CAD build for the part. Positions are in the model's coordinates, mm. A direction names the side the tool comes from. Round coordinates to 2 decimals unless told otherwise and drop trailing zeros. Write each loop counter-clockwise with the first axis right and the second up, starting at its lowest first coordinate (ties: lowest second). Pieces come first, ordered by that corner, then holes. Notation, with made-up numbers: (7.5, -27) -> (45.5, -27) arc R9 ccw to (45.5, -22) -> close; hole circle Ø4 at (-17, -33). An arc over 180 degrees is marked (long way). Put each result on its own line as item: value. Start each with the question number.
1. 3-axis set-ups, long thin cutter, end or side, ignore diameter. For faces 1 (the flat face through (10, -8, 1)), 2 (the flat face through (-10, 8, 1)), 3 (the flat face through (-10, -8, 1)): which of +Z, -Z, +X, -X, +Y, -Y reach the whole face in a straight line?
2. Drill centre lines: line 1 (Z direction, x = 9.75, y = 7.8); line 2 (X direction, y = 9.5, z = 8); line 3 (Z direction, x = -8.75, y = -10.5). Where is each one in solid material? Low to high. Write a range as from..to.
3. Saw through at C-C on z = 7.5. List the corners of the cut face in (x, y).
4. Flat gauge pins, fed straight in: P1, Ø0.6, axis at y = 7, z = 1, coming from the +X side; P2, Ø0.8, axis at y = 10, z = 7, coming from the -X side; P3, Ø3.5, axis at x = 11.5, y = 0, coming from the -Z side; P4, Ø4.5, axis at x = -2.5, z = 7, coming from the +Y side. Where does each tip first touch, or does it go through?
5. Saw through at D-D on x = 5. List the corners of the cut face in (y, z), and give its area (3 significant figures).
6. Saw through at A-A on y = 8.3. List the corners of the cut face in (x, z), and give its area (3 significant figures).
7. Saw through at B-B on x = -11.5. List the corners of the cut face in (y, z), and give its area (3 significant figures).
8. Pull direction Y, two halves, no side cores. Call faces 4 (the flat face through (-3, 10.8, 9)), 5 (the flat face through (2, 8, 16)), 6 (the cylindrical face through (10, 0, 1)), 7 (the cylindrical face through (-13, 0, 1)): pulls with the +Y half, pulls with the -Y half, needs draft (parallel to the pull), parting line crosses it, or undercut.
Autodesk Inventor part; units mm, degrees
ref_plane "YZ Plane" through (0, 0, 0) normal (1, 0, 0) x (0, 1, 0)
ref_plane "XZ Plane" through (0, 0, 0) normal (0, 1, 0) x (-1, 0, 0)
ref_plane "XY Plane" through (0, 0, 0) normal (0, 0, 1) x (1, 0, 0)
sketch "Sketch1" plane through (0, 0, 0) normal (0, 0, 1) x (1, 0, 0)
  line L0 (0, 10.45) -> (0, -10.45)
  arc A0 (10, 10.45) -> (-10, 10.45) centre (0, 10.45) ccw
  arc A1 (-10, -10.45) -> (10, -10.45) centre (0, -10.45) ccw
  line L1 (-10, 10.45) -> (-10, -10.45)
  line L2 (10, 10.45) -> (10, -10.45)
  point P0 (0, 0)
  point P1 (0, 0)
  dimension "d0" = 20.9
  dimension "d3" = 10
  dimension "d4" = 10
extrude "Extrusion1" add sketch "Sketch1" along normal blind 2
sketch "Sketch2" plane through (0, 0, 2) normal (0, 0, 1) x (1, 0, 0)
  line L0 (-10, 10.45) -> (-10, -10.45)
  arc A0 (-10, -10.45) -> (10, -10.45) centre (0, -10.45) ccw
  line L1 (10, -10.45) -> (10, 10.45)
  arc A1 (10, 10.45) -> (-10, 10.45) centre (0, 10.45) ccw
  line L2 (-11.5, 0) -> (11.5, 0)
  circle A2 centre (-11.5, 0) radius 1.5
  circle A3 centre (11.5, 0) radius 1.5
  circle A4 centre (-11.5, 0) radius 2.5
  circle A5 centre (11.5, 0) radius 2.5
  point P0 (0, 0)
  point P1 (0, 0)
  dimension "d7" = 23
  dimension "d8" = 3
  dimension "d9" = 3
  dimension "d10" = 5
  dimension "d11" = 5
extrude "Extrusion2" add sketch "Sketch2" against normal blind 2 contours A4 L2 L0 | L0 A4 | L2 A4 L0 | A5 L1 | L1 L2 A5 | L2 L1 A5
fillet "Fillet1" radius 2.5 4 edges at (10, 2, 1) (10, -2, 1) (-10, 2, 1) (-10, -2, 1)
sketch "Sketch3" plane through (0, 0, 2) normal (0, 0, 1) x (1, 0, 0)
  circle A0 centre (11.5, 0) radius 1.5
  arc A1 (12, -2.4495) -> (12, 2.4495) centre (11.5, 0) ccw
  arc A2 (10, 4.899) -> (12, 2.4495) centre (12.5, 4.899) ccw
  line L0 (10, 4.899) -> (10, 10.45)
  arc A3 (10, 10.45) -> (-10, 10.45) centre (0, 10.45) ccw
  line L1 (-10, 10.45) -> (-10, 4.899)
  arc A4 (-12, 2.4495) -> (-10, 4.899) centre (-12.5, 4.899) ccw
  arc A5 (-12, 2.4495) -> (-12, -2.4495) centre (-11.5, 0) ccw
  arc A6 (-10, -4.899) -> (-12, -2.4495) centre (-12.5, -4.899) ccw
  line L2 (-10, -4.899) -> (-10, -10.45)
  arc A7 (-10, -10.45) -> (10, -10.45) centre (0, -10.45) ccw
  line L3 (10, -10.45) -> (10, -4.899)
  arc A8 (12, -2.4495) -> (10, -4.899) centre (12.5, -4.899) ccw
  circle A9 centre (-11.5, 0) radius 1.5
  line L4 (-6.25, 10.8) -> (-6.25, 5.8)
  line L5 (-6.25, 5.8) -> (6.25, 5.8)
  line L6 (6.25, 5.8) -> (6.25, 10.8)
  line L7 (11.5, 0) -> (0, 0)
  line L8 (0, 0) -> (5.75, 0)
  line L9 (-6.25, 10.8) -> (6.25, 10.8)
  point P0 (0, 0)
  point P1 (0, 10.45)
  dimension "d20" = 5.8
  dimension "d21" = 5
  dimension "d22" = 5
extrude "Extrusion3" add sketch "Sketch3" along normal blind 14 contours L9 L6 L5 L4
sketch "Sketch4" plane through (0, 0, 16) normal (0, 0, 1) x (1, 0, 0)
  line L0 (-6.25, 5.8) -> (6.25, 5.8)
  line L1 (6.25, 5.8) -> (6.25, 10.8)
  line L2 (6.25, 10.8) -> (-6.25, 10.8)
  line L3 (-6.25, 10.8) -> (-6.25, 5.8)
  line L4 (-0.5, 10.8) -> (0.5, 10.8)
  line L5 (6.25, 10.8) -> (-6.25, 10.8)
  arc A0 (-0.5, 9.166) -> (0.5, 9.166) centre (0, 8.3) ccw
  line L6 (-0.5, 10.8) -> (-0.5, 9.166)
  line L7 (0.5, 10.8) -> (0.5, 9.166)
  point P0 (0, 0)
  point P1 (0, 10.8)
  point P2 (0, 10.8)
  dimension "d25" = 1
  dimension "d27" = 2
extrude "Extrusion4" cut sketch "Sketch4" against normal blind 14 contours L2 L7 A0 L6
sketch "Sketch5" plane through (-6.25, 5.8, 2) normal (0, -1, 0) x (1, 0, 0)
  line L0 (12.5, 0) -> (0, 0)
  line L1 (12.5, 0) -> (12.5, 14)
  line L2 (0, 14) -> (12.5, 14)
  line L3 (0, 0) -> (0, 14)
  line L4 (12.5, 0) -> (12.5, 14)
  line L5 (12.5, 14) -> (16, 14)
  circle A0 centre (16, 11.5) radius 2.5
  circle A1 centre (16, 11.5) radius 1.75
  line L6 (16, 9) -> (12.5, 9)
  point P0 (6.25, -2)
  dimension "d30" = 3.5
  dimension "d33" = 3.5
extrude "Extrusion5" add sketch "Sketch5" against normal blind 5 contours L1 L5 A0 L6 | A0
properties part number "Base de la pinza 2"
Return value:
1. face 1: +Z, -Z, +X, -Y
1. face 2: +Z, -Z, -X, +Y
1. face 3: +Z, -Z, -X, -Y
2. line 1: z = 0..2, 11..11.75, 15.25..16
2. line 2: x = -6.25..-0.5, 0.5..6.25
2. line 3: z = 0..2
3. outline: (-6.25, 5.8) -> (6.25, 5.8) -> (6.25, 10.8) -> (0.5, 10.8) -> (0.5, 9.17) arc R1 cw (long way) to (-0.5, 9.17) -> (-0.5, 10.8) -> (-6.25, 10.8) -> close
4. P1: stops at x = 10
4. P2: stops at x = -6.25
4. P3: stops at z = 0
4. P4: stops at y = 10.8
5. outline: (-19.11, 0) -> (19.11, 0) -> (19.11, 2) -> (10.8, 2) -> (10.8, 16) -> (5.8, 16) -> (5.8, 2) -> (-19.11, 2) -> close
5. area: 146 mm^2
6. outline: (-10, 0) -> (10, 0) -> (10, 2) -> (6.25, 2) -> (6.25, 11) -> (9.75, 11) arc R2.5 ccw to (9.75, 16) -> (1, 16) -> (1, 2) -> (-1, 2) -> (-1, 16) -> (-6.25, 16) -> (-6.25, 2) -> (-10, 2) -> close; hole circle Ø3.5 at (9.75, 13.5)
6. area: 205 mm^2
7. outline: (-2.61, 0) -> (-1.5, 0) -> (-1.5, 2) -> (-2.61, 2) -> close; (1.5, 0) -> (2.61, 0) -> (2.61, 2) -> (1.5, 2) -> close
7. area: 4.43 mm^2
8. face 4: pulls with the +Y half
8. face 5: needs draft
8. face 6: undercut
8. face 7: undercut
